Here's how the part is built. I have some questions about the finished solid (model axes, mm). Round coordinates to 2 decimals unless told otherwise and drop trailing zeros. Loops run counter-clockwise (first coordinate to the right, second up) from the corner with the lowest first, then second, coordinate; pieces in that order, holes last. Notation, with made-up numbers: M 29,88.25 L 65,88.25 A17 ccw 65,116.25 Z; hole C 16,14.25 d7. An arc over 180 degrees is marked long. Use a Markdown table: item, result.
from build123d import *

# Parameters (mm, degrees)
F0_R            = 2.65
F0_R_2          = 3.75
F0_R_3          = 1.6
F0_R_4          = 3
F1_DEPTH        = 10
F2_D            = 5.5
F2_CSINK_D      = 11.2
F2_CSINK_ANGLE  = 90
F3_D            = 5.5
F3_CBORE_D      = 22.1
F3_CBORE_DEPTH  = 2.1
F4_DEPTH        = 10.001
F5_D            = 3.3
F5_CBORE_D      = 6.5
F5_CBORE_DEPTH  = 3
F6_D            = 7.5
F6_CBORE_D      = 11.75
F6_CBORE_DEPTH  = 5
F9_D            = 3.3
F9_CBORE_D      = 6.5
F9_CBORE_DEPTH  = 3
F10_D           = 5.5
F10_CBORE_D     = 9.75
F10_CBORE_DEPTH = 5
F12_DEPTH       = 25
F13_R           = 5


with BuildPart() as f1:
    # F0 (on Top) → F1 (new body)
    with BuildSketch(Plane.XY):
        Polygon((-125, -55), (125, -55), (125, 55), (-125, 55), (-125, 28), (-97, 0), (-125, -28), align=None)
        with Locations((-105, -45)):
            Circle(F0_R, mode=Mode.SUBTRACT)
        with Locations((-25.3, -45)):
            Circle(F0_R_2, mode=Mode.SUBTRACT)
        with Locations((22.0002193564, -15.4997806436)):
            Circle(F0_R_3, mode=Mode.SUBTRACT)
        with Locations((52.9997806436, -15.4997806436)):
            Circle(F0_R_3, mode=Mode.SUBTRACT)
        with Locations((-105, 45)):
            Circle(F0_R, mode=Mode.SUBTRACT)
        with Locations((-25.3, 45)):
            Circle(F0_R_2, mode=Mode.SUBTRACT)
        with Locations((37.5, 0)):
            Circle(F0_R_4, mode=Mode.SUBTRACT)
        with Locations((22.0002193564, 15.4997806436)):
            Circle(F0_R_3, mode=Mode.SUBTRACT)
        with Locations((52.9997806436, 15.4997806436)):
            Circle(F0_R_3, mode=Mode.SUBTRACT)
        with Locations((75, 0)):
            Circle(F0_R, mode=Mode.SUBTRACT)
        with Locations((95, 0)):
            Circle(F0_R, mode=Mode.SUBTRACT)
        with Locations((115, 0)):
            Circle(F0_R, mode=Mode.SUBTRACT)
        with Locations((75, 35)):
            Circle(F0_R_3, mode=Mode.SUBTRACT)
        with Locations((85, 35)):
            Circle(F0_R_3, mode=Mode.SUBTRACT)
        Polygon((-125, 28), (-125, -28), (-97, 0), align=None)
    extrude(amount=F1_DEPTH)

    # F2 (through all)
    with Locations(Plane(origin=(0, 0, 0), x_dir=(1, 0, 0), z_dir=(0, 0, -1))):
        with Locations((75, 0), (95, 0), (115, 0)):
            CounterSinkHole(F2_D / 2, F2_CSINK_D / 2, counter_sink_angle=F2_CSINK_ANGLE)

    # F3 (through all)
    with Locations(Plane(origin=(0, 0, 0), x_dir=(1, 0, 0), z_dir=(0, 0, -1))):
        with Locations((37.5, 0)):
            CounterBoreHole(F3_D / 2, F3_CBORE_D / 2, F3_CBORE_DEPTH)

    # F0 (on Top) → F4 (cut, through all)
    with BuildSketch(Plane.XY):
        Polygon((-125, 28), (-125, -28), (-97, 0), align=None)
    extrude(amount=F4_DEPTH, mode=Mode.SUBTRACT)

    # F5 (through all)
    with Locations(Plane(origin=(0, 0, 0), x_dir=(1, 0, 0), z_dir=(0, 0, -1))):
        with Locations((75, -35), (85, -35)):
            CounterBoreHole(F5_D / 2, F5_CBORE_D / 2, F5_CBORE_DEPTH)

    # F6 (through all)
    with Locations(Plane(origin=(0, 0, 0), x_dir=(1, 0, 0), z_dir=(0, 0, -1))):
        with Locations((-25.3, 45), (-25.3, -45)):
            CounterBoreHole(F6_D / 2, F6_CBORE_D / 2, F6_CBORE_DEPTH)

    # F9 (through all)
    with Locations(Plane.XY.offset(10)):
        with Locations((52.9997806436, 15.4997806436), (52.9997806436, -15.4997806436), (22.0002193564, -15.4997806436), (22.0002193564, 15.4997806436)):
            CounterBoreHole(F9_D / 2, F9_CBORE_D / 2, F9_CBORE_DEPTH)

    # F10 (through all)
    with Locations(Plane(origin=(0, 0, 0), x_dir=(1, 0, 0), z_dir=(0, 0, -1))):
        with Locations((-105, 45), (-105, -45)):
            CounterBoreHole(F10_D / 2, F10_CBORE_D / 2, F10_CBORE_DEPTH)

    # F11 (on offset) → F12 (cut)
    with BuildSketch(Plane.XY.offset(10)):
        Polygon((125, 55), (-10.3, 55), (24.1719999404, 26.0745575641), (60, 26.0745575641), (70.8289389059, 44.8308299412), (89.1710610941, 44.8308299412), (100, 26.0745575641), (125, 26.0745575641), align=None)
        Polygon((125, -55), (125, -26.0745575641), (24.1719999404, -26.0745575641), (-10.3, -55), align=None)
        Polygon((-65.8571067812, -26.8935335215), (-93.9635732597, -55), (-37.7506403027, -55), align=None)
        Polygon((-37.7506403027, 55), (-93.9635732597, 55), (-65.8571067812, 26.8935335215), align=None)
    extrude(amount=-F12_DEPTH, mode=Mode.SUBTRACT)

    # F13
    f13_edges = [f1.edges().sort_by_distance(p)[0] for p in [
        (-125, -28, 5),
        (-125, -55, 5),
        (-125, 28, 5),
        (-125, 55, 5),
        (24.172, -26.074558, 5),
        (-10.3, -55, 5),
        (125, -26.074558, 5),
        (125, 26.074558, 5),
        (100, 26.074558, 5),
        (89.171061, 44.83083, 5),
        (70.828939, 44.83083, 5),
        (60, 26.074558, 5),
        (24.172, 26.074558, 5),
        (-10.3, 55, 5),
        (-65.857107, -26.893534, 5),
        (-65.857107, 26.893534, 5),
        (-93.963573, -55, 5),
        (-37.75064, -55, 5),
        (-37.75064, 55, 5),
        (-93.963573, 55, 5),
    ]]
    fillet(f13_edges, radius=F13_R)


solid = f1.part
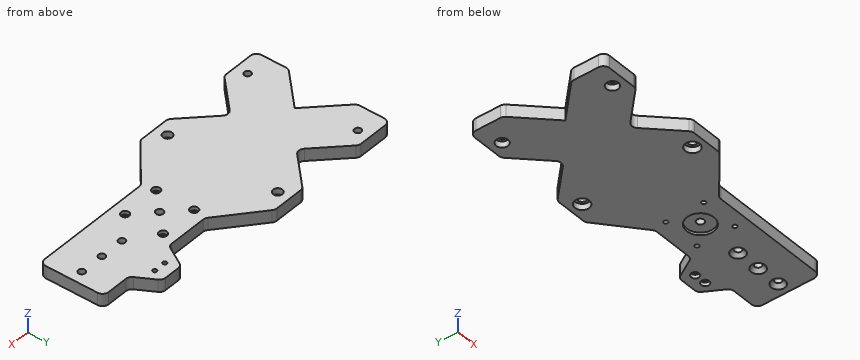
1. Imagine slicing it at B-B, the plane z = 8.5. State how many separate pieces and enclosed holes the cut face has, then the cut area to 3 significant figures.
Answer sheet:
| item | result |
|---|---|
| separate pieces | 1 |
| enclosed holes | 14 |
| area | 18,500 mm2 |
2. Imagine slicing it at D-D, the plane x = -79. Write out the boundary of the cut face in (y, z).
Answer sheet:
| item | result |
|---|---|
| outline | M -40.04,0 L 40.04,0 L 40.04,10 L -40.04,10 Z |
3. Imagine slicing it at C-C, the plane x = 44. Write out the boundary of the cut face in (y, z).
Answer sheet:
| item | result |
|---|---|
| outline | M -26.07,0 L -8.94,0 L -8.94,2.1 L 8.94,2.1 L 8.94,0 L 26.07,0 L 26.07,10 L -26.07,10 Z |
4. Imagine slicing it at A-A, the plane x = 115. Write out the boundary of the cut face in (y, z).
Answer sheet:
| item | result |
|---|---|
| outline | M -26.07,0 L -5.6,0 L -2.75,2.85 L -2.75,10 L -26.07,10 Z; M 2.75,2.85 L 5.6,0 L 26.07,0 L 26.07,10 L 2.75,10 Z |
5. For pin 1 Ø2 at (x, z) = (42, 9) entering from -Y; pin 2 Ø5 at (y, z) = (41.5, 4.5) entering from +X; pin 3 Ø3 at (x, y) = (84.5, 36.5) entering from -Z; pin 4 Ø2 at (x, y) = (85, 35) entering from +Z, each with a flat end and sliding along its axis, tell me the tip position at first contact or that it passes through.
Answer sheet:
| item | result |
|---|---|
| pin 1 | y = -26.07 |
| pin 2 | x = 92.54 |
| pin 3 | z = 3 |
| pin 4 | through |
6. I need wall thicknesses on probe 1 along X at (y, z) = (-46, 1.75); probe 2 along X at (y, z) = (45, 3.95) (3 decimals); probe 3 along X at (y, z) = (33, 5). Which ranges of each line are inside material? Lowest first, please. Write a range as from..to.
Answer sheet:
| item | result |
|---|---|
| probe 1 | -125..-109.77, -100.23..-84.96, -46.75..-31.09, -19.51..0.43 |
| probe 2 | -125..-109.875, -100.125..-83.964, -47.751..-31.175, -19.425..1.618 |
| probe 3 | -125..-71.96, -59.75..15.92, 64..96 |
